The listing builds one solid part. Answer for the finished solid, in the listing's coordinates (mm). Face numbers are marked on the shaded views. A direction names the side the tool comes from. Coordinates: 2 decimals unless noted, no trailing zeros. Write each loop counter-clockwise with the first axis right and the second up, starting at its lowest first coordinate (ties: lowest second). Pieces come first, ordered by that corner, then holes. Notation, with made-up numbers: M 68.25,69 L 88.25,69 A34 ccw 88.25,101 Z; hole C 50,-10 d5. An arc over 180 degrees is marked long. Answer as a JSON object with one key per item and string values. Group by question number.
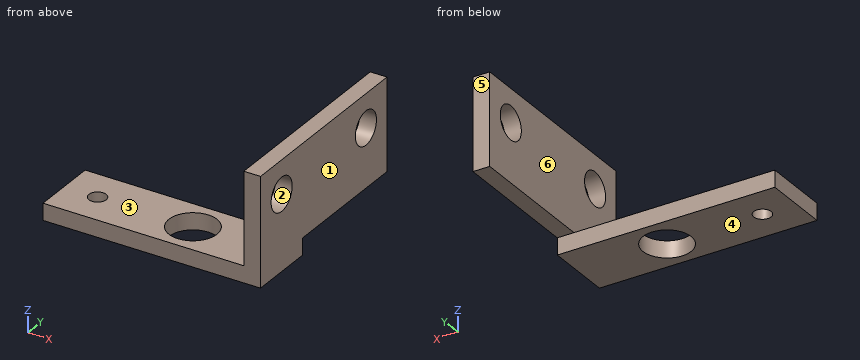
from build123d import *

# Parameters (mm, degrees)
SKETCH1_W           = 82.55
SKETCH1_H           = 25.4
BOSS_EXTRUDE1_DEPTH = 6.35
SKETCH2_W           = 6.35
SKETCH2_H           = 25.4
BOSS_EXTRUDE2_DEPTH = 34.925
SKETCH4_R           = 6.35
CUT_EXTRUDE1_DEPTH  = 96.725065291
SKETCH5_R           = 3.302
SKETCH5_R_2         = 9.144
CUT_EXTRUDE2_DEPTH  = 38.1
SKETCH6_W           = 6.35
SKETCH6_H           = 34.925
BOSS_EXTRUDE3_DEPTH = 50.8
SKETCH7_R           = 6.35
CUT_EXTRUDE3_DEPTH  = 120.685287839


with BuildPart() as part:
    # Sketch1 → Boss-Extrude1 (new body)
    with BuildSketch(Plane.XY):
        with Locations((41.275, 12.7)):
            Rectangle(SKETCH1_W, SKETCH1_H)
    extrude(amount=BOSS_EXTRUDE1_DEPTH)

    # Sketch2 → Boss-Extrude2 (add)
    with BuildSketch(Plane.XY.offset(6.35)):
        with Locations((79.375, 12.7)):
            Rectangle(SKETCH2_W, SKETCH2_H)
    extrude(amount=BOSS_EXTRUDE2_DEPTH)

    # Sketch4 → Cut-Extrude1 (cut, through all)
    with BuildSketch(Plane(origin=(82.55, 0, 0), x_dir=(0, 0, -1), z_dir=(1, 0, 0))):
        with Locations((-28.575, 12.7)):
            Circle(SKETCH4_R)
    extrude(amount=-CUT_EXTRUDE1_DEPTH, mode=Mode.SUBTRACT)

    # Sketch5 → Cut-Extrude2 (cut)
    with BuildSketch(Plane.XY.offset(6.35)):
        with Locations((12.7, 12.7)):
            Circle(SKETCH5_R)
        with Locations((48.895, 12.7)):
            Circle(SKETCH5_R_2)
    extrude(amount=-CUT_EXTRUDE2_DEPTH, mode=Mode.SUBTRACT)

    # Sketch6 → Boss-Extrude3 (add)
    with BuildSketch(Plane(origin=(0, 25.4, 0), x_dir=(1, 0, 0), z_dir=(0, 1, 0))):
        with Locations((79.375, -23.8125)):
            Rectangle(SKETCH6_W, SKETCH6_H)
    extrude(amount=BOSS_EXTRUDE3_DEPTH)

    # Sketch7 → Cut-Extrude3 (cut, through all)
    with BuildSketch(Plane(origin=(82.55, 0, 0), x_dir=(0, 0, -1), z_dir=(1, 0, 0))):
        with Locations((-28.575, 63.5)):
            Circle(SKETCH7_R)
    extrude(amount=-CUT_EXTRUDE3_DEPTH, mode=Mode.SUBTRACT)


solid = part.part
Item 1: A cutting plane is placed at D-D, the plane y = 12.7. Write down the section's boundary in (x, z) (3 decimals), and give its area (3 significant figures).
Item 2: Consider L1, parallel to Z at x = 77, y = 63 (3 decimals); L2, parallel to X at y = 44.5, z = 22; L3, parallel to Y at x = 12.7, z = 3.75. Determine where each line is inside the solid, lowest interval first. Write a range as from..to.
Item 3: A tool of negligible diameter and unlimited length cuts with its end or side. For the marked faces 5 and 6, from which of +Z, -Z, +X, -X, +Y, -Y can it reach the whole face along a straight path? Write none if from no direction.
Item 4: A cutting plane is placed at C-C, the plane z = 30.5. Write down the section's boundary in (x, y), and give its area (3 significant figures).
Item 5: For a pull along Z with two mould halves and no side action, classify the marked faces 1, 2, 3 and 4 as +Z half, -Z half, draft (parallel to the pull), parting line (faces both ways), or undercut.
Item 6: A cutting plane is placed at A-A, the plane y = 63.5. Write down the section's boundary in (x, z) (3 decimals), and give its area (3 significant figures).
Item 7: Flat-ended cylindrical pins translate along their axes: pin 1 Ø6 at (x, y) = (12.7, 12.7) entering from +Z; pin 2 Ø6 at (y, z) = (8, 21.5) entering from -X; pin 3 Ø7 at (x, z) = (44, 3.5) entering from +Y; pin 4 Ø20.5 at (x, y) = (21, 14) entering from +Z. Find the tip coordinate at first contact, or state that the pin passes through.
Item 8: A cutting plane is placed at B-B, the plane x = 12.7. Write down the section's boundary in (y, z), and give its area (3 significant figures).
Answer:
{
 "1": {"outline": "M 0,0 L 9.398,0 L 9.398,6.35 L 0,6.35 Z; M 16.002,0 L 39.751,0 L 39.751,6.35 L 16.002,6.35 Z; M 58.039,0 L 82.55,0 L 82.55,22.225 L 76.2,22.225 L 76.2,6.35 L 58.039,6.35 Z; M 76.2,34.925 L 82.55,34.925 L 82.55,41.275 L 76.2,41.275 Z", "area": "507 mm2"},
 "2": {"L1": "6.35..22.245, 34.905..41.275", "L2": "76.2..82.55", "L3": "0..9.4, 16..25.4"},
 "3": {"face 5": "+Z, -Z, +X, -X, +Y", "face 6": "+Z, -X, +Y, -Y"},
 "4": {"outline": "M 76.2,0 L 82.55,0 L 82.55,6.65 L 76.2,6.65 Z; M 76.2,18.75 L 82.55,18.75 L 82.55,57.45 L 76.2,57.45 Z; M 76.2,69.55 L 82.55,69.55 L 82.55,76.2 L 76.2,76.2 Z", "area": "330 mm2"},
 "5": {"face 1": "draft", "face 2": "undercut", "face 3": "+Z half", "face 4": "-Z half"},
 "6": {"outline": "M 76.2,6.35 L 82.55,6.35 L 82.55,22.225 L 76.2,22.225 Z; M 76.2,34.925 L 82.55,34.925 L 82.55,41.275 L 76.2,41.275 Z", "area": "141 mm2"},
 "7": {"pin 1": "through", "pin 2": "x = 76.2", "pin 3": "y = 25.4", "pin 4": "z = 6.35"},
 "8": {"outline": "M 0,0 L 9.4,0 L 9.4,6.35 L 0,6.35 Z; M 16,0 L 25.4,0 L 25.4,6.35 L 16,6.35 Z", "area": "119 mm2"}
}
